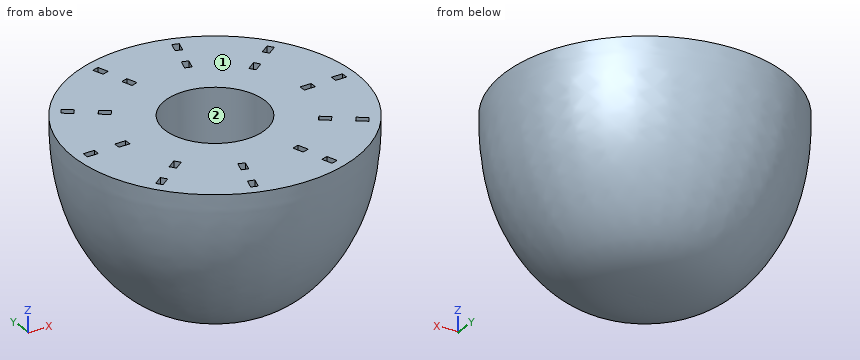
from build123d import *

# Parameters (mm, degrees)
F2_R     = 22.5
F3_DEPTH = 70
F4_W     = 5
F4_H     = 3
F5_DEPTH = 6


with BuildPart() as f1:
    # F0 (on Front) → F1 (revolve)
    with BuildSketch(Plane.XZ):
        with BuildLine():
            Line((63.5, 0), (0, 0))
            Line((0, 0), (0, -80))
            add(Edge.make_bspline(
                [(0, -80), (10.2409981191, -80.0559148192), (34.8220828583, -78.7447738141), (62.2798344564, -39.0297563597), (63.5, -9.5845087473), (63.5, 0)],
                knots=[0, 0, 0, 0, 0.3058329124, 0.6687596422, 1, 1, 1, 1], degree=3))
        make_face()
    revolve(axis=Axis((0, 0, -40), (0, 0, -1)))

    # F2 (on face) → F3 (cut)
    with BuildSketch(Plane.XY):
        Circle(F2_R)
    extrude(amount=-F3_DEPTH, mode=Mode.SUBTRACT)

    # F4 (on Top) → F5 (cut)
    with BuildSketch(Plane.XY):
        with Locations((-42.125, 0)):
            Rectangle(F4_W, F4_H)
        with Locations((-56.375, 0)):
            Rectangle(F4_W, F4_H)
        Polygon((-46.7491976654, -35.8193822203), (-42.7041126935, -32.8804559588), (-44.4674684504, -30.4534049757), (-48.5125534223, -33.3923312372), align=None)
        Polygon((-31.1756205237, -24.5045161137), (-32.9389762805, -22.0774651305), (-36.9840612524, -25.016391392), (-35.2207054955, -27.4434423751), align=None)
        Polygon((-16.7667907694, -56.4569778884), (-15.2217057975, -51.701695307), (-18.0748753464, -50.7746443238), (-19.6199603183, -55.5299269053), align=None)
        Polygon((-10.8182136277, -38.1491399498), (-13.6713831766, -37.2220889666), (-15.2164681484, -41.9773715481), (-12.3632985995, -42.9044225312), align=None)
        Polygon((19.6199603183, -55.5299269053), (18.0748753464, -50.7746443238), (15.2217057975, -51.701695307), (16.7667907694, -56.4569778884), align=None)
        Polygon((13.6713831766, -37.2220889666), (10.8182136277, -38.1491399498), (12.3632985995, -42.9044225312), (15.2164681484, -41.9773715481), align=None)
        Polygon((48.5125534223, -33.3923312372), (44.4674684504, -30.4534049757), (42.7041126935, -32.8804559588), (46.7491976654, -35.8193822203), align=None)
        Polygon((32.9389762805, -22.0774651305), (31.1756205237, -24.5045161137), (35.2207054955, -27.4434423751), (36.9840612524, -25.016391392), align=None)
        with Locations((56.375, 0)):
            Rectangle(F4_W, F4_H)
        with Locations((42.125, 0)):
            Rectangle(F4_W, F4_H)
        Polygon((46.7491976654, 35.8193822203), (42.7041126935, 32.8804559588), (44.4674684504, 30.4534049757), (48.5125534223, 33.3923312372), align=None)
        Polygon((31.1756205237, 24.5045161137), (32.9389762805, 22.0774651305), (36.9840612524, 25.016391392), (35.2207054955, 27.4434423751), align=None)
        Polygon((16.7667907694, 56.4569778884), (15.2217057975, 51.701695307), (18.0748753464, 50.7746443238), (19.6199603183, 55.5299269053), align=None)
        Polygon((10.8182136277, 38.1491399498), (13.6713831766, 37.2220889666), (15.2164681484, 41.9773715481), (12.3632985995, 42.9044225312), align=None)
        Polygon((-19.6199603183, 55.5299269053), (-18.0748753464, 50.7746443238), (-15.2217057975, 51.701695307), (-16.7667907694, 56.4569778884), align=None)
        Polygon((-13.6713831766, 37.2220889666), (-10.8182136277, 38.1491399498), (-12.3632985995, 42.9044225312), (-15.2164681484, 41.9773715481), align=None)
        Polygon((-48.5125534223, 33.3923312372), (-44.4674684504, 30.4534049757), (-42.7041126935, 32.8804559588), (-46.7491976654, 35.8193822203), align=None)
        Polygon((-32.9389762805, 22.0774651305), (-31.1756205237, 24.5045161137), (-35.2207054955, 27.4434423751), (-36.9840612524, 25.016391392), align=None)
    extrude(amount=-F5_DEPTH, mode=Mode.SUBTRACT)


solid = f1.part
Can you work these out from the model? Positions are in its coordinate system, mm. Face numbers are marked on the shaded views. Give positions to 0.01 mm unless a question says otherwise; leave off trailing zeros. One line per question, with ' | ' between items.
Item 1: I'm going to push flat-ended pins straight in: pin 1 Ø1.5 at (y, z) = (0, -3) entering from +X; pin 2 Ø0.9 at (x, y) = (-41, 0) entering from +Z; pin 3 Ø2.5 at (x, z) = (41.5, -4) entering from +Y; pin 4 Ø10 at (y, z) = (-48.5, -68) entering from +X. Where does each tip first touch, or does it pass through?
Answer block:
pin 1: stops at x = 63.49 | pin 2: stops at z = -6 | pin 3: stops at y = 49.07 | pin 4: passes through
Item 2: We'd pull the mould along Y, two halves only. Please class the marked faces 1 and 2: released by +Y, released by -Y, zero draft, split by the parting line, or undercut.
Answer block:
face 1: zero draft | face 2: undercut
Item 3: Please list where these lines run through material, in increasing order: L1, parallel to X at y = -19.5, z = -66; L2, parallel to Y at x = 0, z = -17; L3, parallel to Z at x = -9.5, y = -49.5.
Answer block:
L1: x = -36.01 to -11.22, 11.22 to 36.01 | L2: y = -62.64 to -22.5, 22.5 to 62.64 | L3: z = -53.87 to 0
